Autodesk Inventor part; units mm, degrees
ref_plane "YZ Plane" through (0, 0, 0) normal (1, 0, 0) x (0, 1, 0)
ref_plane "XZ Plane" through (0, 0, 0) normal (0, 1, 0) x (-1, 0, 0)
ref_plane "XY Plane" through (0, 0, 0) normal (0, 0, 1) x (1, 0, 0)
sketch "Sketch1" plane through (0, 0, 0) normal (0, 0, 1) x (1, 0, 0)
  circle A0 centre (-3.1769, 113.7672) radius 2.0955
  circle A1 centre (-3.1769, -102.1328) radius 2.0955
  line L0 (-9.5269, 120.1172) -> (4.5684, 120.1172)
  line L1 (-9.5269, -121.1828) -> (-9.5269, 120.1172)
  line L2 (-9.5269, 120.1172) -> (-58.0591, 120.1172)
  line L3 (-79.3769, 60.3213) -> (-79.3769, -95.7828)
  line L4 (-9.5269, -121.1828) -> (-9.5269, 120.1172)
  line L5 (-61.0624, 117.9719) -> (-78.0039, 68.5592)
  arc A2 (-78.0039, 68.5592) -> (-79.3769, 60.3213) centre (-53.9769, 60.3213) ccw
  arc A3 (-79.3769, -95.7828) -> (-53.9769, -121.1828) centre (-53.9769, -95.7828) ccw
  arc A4 (-58.0591, 120.1172) -> (-61.0624, 117.9719) centre (-58.0591, 116.9422) ccw
  arc A5 (22.9235, 106.1658) -> (4.5684, 120.1172) centre (4.5684, 101.0672) ccw
  arc A6 (22.2231, -121.1828) -> (26.6067, -107.95) centre (14.337, -111.228) ccw
  line L6 (-41.2769, -121.1828) -> (22.2231, -121.1828)
  line L7 (26.6067, -107.95) -> (26.6067, 90.8579)
  line L8 (22.9235, 106.1658) -> (26.6067, 90.8579)
  line L9 (-53.9769, -121.1828) -> (-41.2769, -121.1828)
  point P0 (0, 0)
  point P1 (-79.3769, -121.1828)
  dimension "d0" = 4.191
  dimension "d1" = 4.191
  dimension "d2" = 69.85
  dimension "d3" = 25.4
  dimension "d4" = 3.175
  dimension "d5" = 19.05
  dimension "d16" = 12.7
  dimension "d18" = 63.5
extrude "Extrusion1" add sketch "Sketch1" along normal blind 1.5875
bend part "Bend Part1" radius 9.525 angle 55 line through (-9.5269, -121.1828, 0) along (0, 1, 0) centre toward (0, 0, 1) moving side (-1, 0, 0) both sides no
properties part number "wedge" material "Acetal Resin, White"
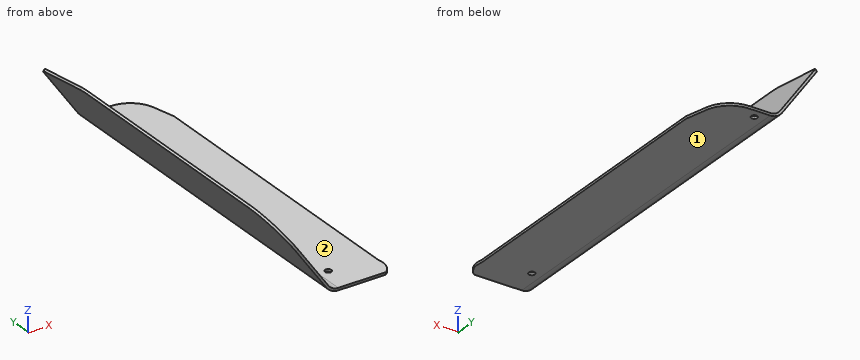
The listing builds one solid part. Answer for the finished solid, in the listing's coordinates (mm). Face numbers are marked on the shaded views. A direction names the side the tool comes from. Coordinates: 2 decimals unless noted, no trailing zeros. Write each loop counter-clockwise with the first axis right and the second up, starting at its lowest first coordinate (ties: lowest second). Pieces come first, ordered by that corner, then holes. Notation, with made-up numbers: (61, -3) - (86, -3) arc R17 ccw to (86, 8) - close; hole circle Ø3 at (70, 75.5). An arc over 180 degrees is marked (long way). Return JSON: item names as keys, results as strings. Group by question number.
1. Which of the six approach directions +Z, -Z, +X, -X, +Y, -Y give full straight-line access (tool end or side, diameter ignored) to the marked faces 1 and 2?
2. Straight lines are drawn through the part: L1, parallel to Z at x = 18, y = -104; L2, parallel to Z at x = -32, y = 74; L3, parallel to X at y = 1, z = 18. For each, find the intervals that lie inside material, in ascending order.
3. A cutting plane is placed at B-B, the plane z = 27. Determine the outline of the cut face in (x, y), plus the area to 3 significant figures.
4. Given pin 1 (6.5 mm diameter, centred on x = -3.18, y = 113.77, fed in from +Z); pin 2 (4 mm diameter, centred on y = 23, z = 21.5, fed in from +X); pin 3 (2.5 mm diameter, centred on x = -3.18, y = -102.13, fed in from +Z) (1 decimal); pin 4 (2 mm diameter, centred on x = -31.5, y = -92, fed in from -Z), each flat-ended and moving along its own axis, determine where each tip first touches the part or whether it passes through.
5. A cutting plane is placed at D-D, the plane x = 12. Determine the outline of the cut face in (y, z).
Ans:
{
 "1": {"face 1": "-Z, +X, -X, +Y, -Y", "face 2": "+Z, +X, +Y, -Y"},
 "2": {"L1": "0 to 1.59", "L2": "25.01 to 27.78", "L3": "-27.09 to -25.15"},
 "3": {"outline": "(-33.39, -121.18) - (-31.45, -121.18) - (-31.45, 120.12) - (-33.39, 120.12) - close", "area": "468 mm²"},
 "4": {"pin 1": "z = 1.59", "pin 2": "x = -26.2", "pin 3": "through", "pin 4": "z = 22.87"},
 "5": {"outline": "(-121.18, 0) - (118.61, 0) - (118.61, 1.59) - (-121.18, 1.59) - close"}
}
